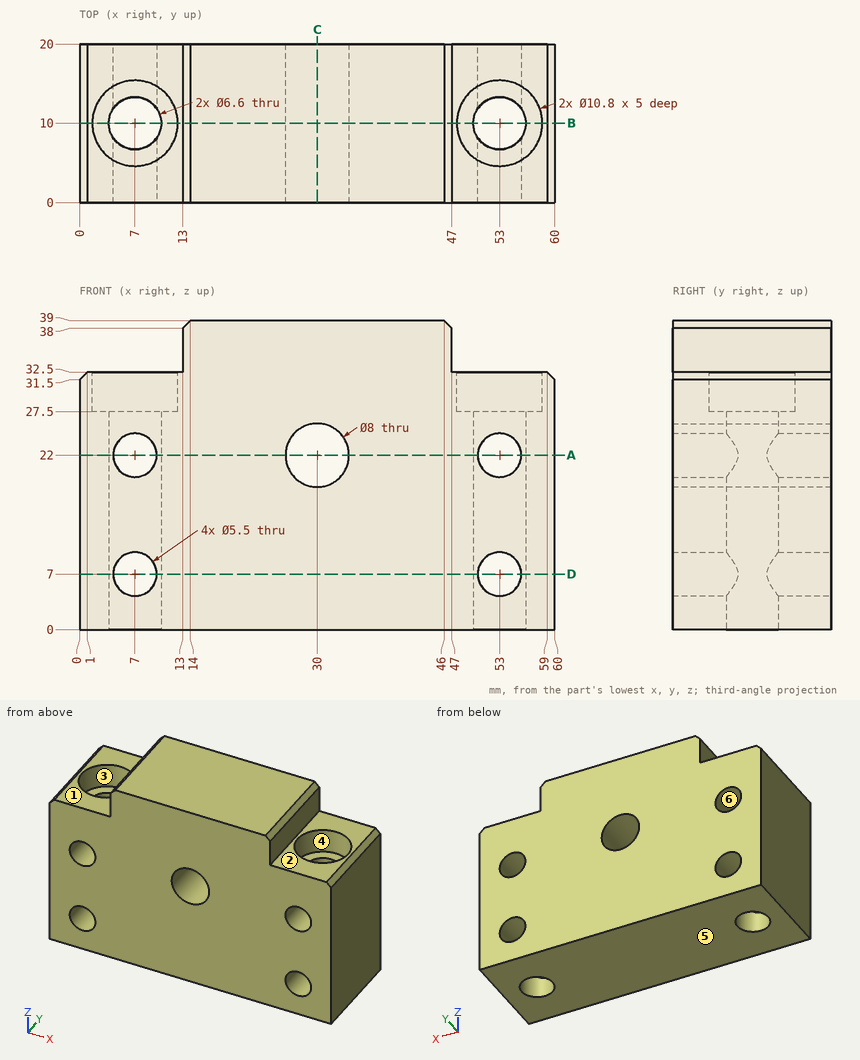
Drawing for the job (mm, zero at the part's lowest x, y, z). A direction names the side the tool comes from. Coordinates: 2 decimals unless noted, no trailing zeros. Loops run counter-clockwise (first coordinate to the right, second up) from the corner with the lowest first, then second, coordinate; pieces in that order, holes last. Notation, with made-up numbers: (75, 49) - (133, 49) arc R30 cw to (133, 77) - close; hole circle Ø7 at (-39, -28.5). An arc over 180 degrees is marked (long way). Return JSON: item names as keys, results as strings.
1. Band-saw the part on D-D (z = 7). Give the cut face in (x, y).
Result:
{"outline": "(0, 0) - (4.25, 0) - (4.25, 8.18) arc R3.3 cw to (4.25, 11.82) - (4.25, 20) - (0, 20) - close; (9.75, 0) - (50.25, 0) - (50.25, 8.18) arc R3.3 cw to (50.25, 11.82) - (50.25, 20) - (9.75, 20) - (9.75, 11.82) arc R3.3 cw to (9.75, 8.18) - close; (55.75, 0) - (60, 0) - (60, 20) - (55.75, 20) - (55.75, 11.82) arc R3.3 cw to (55.75, 8.18) - close"}
2. Band-saw the part on C-C (x = 30). Give the cut face in (y, z), and give its area (3 significant figures).
Result:
{"outline": "(0, 0) - (20, 0) - (20, 18) - (0, 18) - close; (0, 26) - (20, 26) - (20, 39) - (0, 39) - close", "area": "620 mm2"}
3. Band-saw the part on A-A (z = 22). Give the cut face in (x, y).
Result:
{"outline": "(0, 0) - (4.25, 0) - (4.25, 8.18) arc R3.3 cw to (4.25, 11.82) - (4.25, 20) - (0, 20) - close; (9.75, 0) - (26, 0) - (26, 20) - (9.75, 20) - (9.75, 11.82) arc R3.3 cw to (9.75, 8.18) - close; (34, 0) - (50.25, 0) - (50.25, 8.18) arc R3.3 cw to (50.25, 11.82) - (50.25, 20) - (34, 20) - close; (55.75, 0) - (60, 0) - (60, 20) - (55.75, 20) - (55.75, 11.82) arc R3.3 cw to (55.75, 8.18) - close"}
4. Mould opens along Z. For the marked faces 4, 5 and 6 say: released by +Z, released by -Z, zero draft, split by the parting line, or undercut.
Result:
{"face 4": "zero draft", "face 5": "released by -Z", "face 6": "undercut"}
5. 3-axis set-ups, long thin cutter, end or side, ignore diameter. For the marked faces 1, 2 and 3: which of +Z, -Z, +X, -X, +Y, -Y reach the whole face in a straight line?
Result:
{"face 1": "+Z, -X, +Y, -Y", "face 2": "+Z, +X, +Y, -Y", "face 3": "+Z"}
6. Drop flat-ended pins along their axis: pin 1 (12 mm diameter, centred on x = 5, y = 9.5, fed in from +Z); pin 2 (8.5 mm diameter, centred on x = 52.5, y = 9, fed in from +Z); pin 3 (4.5 mm diameter, centred on y = 6.5, z = 34, fed in from +X). Give the stop position or say it passes through.
Result:
{"pin 1": "stops at z = 32.5", "pin 2": "stops at z = 27.5", "pin 3": "stops at x = 59.75"}
7. Probe L1, parallel to Z at x = 53, y = 6.25; L2, parallel to Z at x = 53, y = 2; L3, parallel to Y at x = 53, z = 14. List the from-to ranges inside material, lowest first. Write a range as from..to.
Result:
{"L1": "z = 0..4.25, 9.75..19.25, 24.75..27.5", "L2": "z = 0..4.25, 9.75..19.25, 24.75..32.5", "L3": "y = 0..6.7, 13.3..20"}
8. Band-saw the part on B-B (y = 10). State how many separate pieces and enclosed holes the cut face has, and give its area (3 significant figures).
Result:
{"separate pieces": "3", "enclosed holes": "1", "area": "1,650 mm2"}
